Here's how the part is built. I have some questions about the finished solid (model axes, mm). A direction names the side the tool comes from. Coordinates: 2 decimals unless noted, no trailing zeros. Loops run counter-clockwise (first coordinate to the right, second up) from the corner with the lowest first, then second, coordinate; pieces in that order, holes last. Notation, with made-up numbers: M 42.25,4.5 L 74.25,4.5 A15 ccw 74.25,14.5 Z; hole C 67.25,11.5 d1. An arc over 180 degrees is marked long. Use one line per item in the form item = value. Start each with the question number.
(1) On a 3-axis mill with a long thin cutter (end or side, diameter ignored), from which of +Z, -Z, +X, -X, +Y, -Y can I reach the whole of each face in a straight line? I mean faces 4 (the flat face through (-23, 46, 27)), 5 (the flat face through (-1, 40, 34)), 6 (the flat face through (-26.5, 45, 0)), 7 (the cylindrical face through (-105, 20, -47)). Say none if no direction works.
(2) Imagine slicing it at C-C, the plane x = 46. Please give me the cut outline in (y, z), and give its area (3 significant figures).
(3) Imagine slicing it at A-A, the plane z = 10. Please give me the cut outline in (x, y), and give its area (3 significant figures).
(4) Imagine slicing it at B-B, the plane y = 20. State how many separate pieces and enclosed holes the cut face has, and give its area (3 significant figures).
(5) Will these pins go through, and if not, where does the flat tip stop? P1, Ø2, axis at x = 0, z = 65, coming from the -Y side; P2, Ø5, axis at x = 56.5, z = 16.5, coming from the -Y side; P3, Ø5, axis at y = 20, z = 50, coming from the -X side.
(6) Thinking about a two-plate mould opening in X: for faces 1 (the cylindrical face through (20.997, 42.958, -26.069)), 2 (the flat face through (-110, 24, 1)), 3 (the flat face through (-1, 43, -75)), which applies, +X half, -X half, draft (parallel to the pull), parting line (faces both ways), or undercut?
(7) Please list where these lines run through material, in increasing order: L1, parallel to Z at x = -23, y = 44; L2, parallel to Z at x = -107.5, y = 20; L3, parallel to Z at x = 0, y = 43.
```python
from build123d import *

# Parameters (mm, degrees)
PAD_DEPTH       = 75
SKETCH001_R     = 3
POCKET_DEPTH    = 110.001
FILLET_R        = 3
FILLET001_R     = 1
SKETCH002_R     = 2.1
POCKET001_DEPTH = 6
POCKET002_DEPTH = 10.001
FILLET002_R     = 1
SKETCH004_R     = 1.35
POCKET003_DEPTH = 6


with BuildPart() as part:
    # Sketch → Pad (new body, symmetric)
    with BuildSketch(Plane.XY):
        Polygon((0, 40), (-100, 40), (-100, 0), (-110, 0), (-110, 50), (0, 50), align=None)
        Polygon((0, 40), (0, 50), align=None)
    extrude(amount=PAD_DEPTH, both=True)

    # Sketch001 (on Face3 of Pad) → Pocket (cut, through all)
    with BuildSketch(Plane(origin=(-110, 0, 0), x_dir=(0, -1, 0), z_dir=(-1, 0, 0))):
        with Locations((-20, -50)):
            Circle(SKETCH001_R)
        with Locations((-20, 50)):
            Circle(SKETCH001_R)
    extrude(amount=-POCKET_DEPTH, mode=Mode.SUBTRACT)

    # Fillet
    fillet_edges = [part.edges().sort_by_distance(p)[0] for p in [
        (-105, 0, -75),
        (-100, 40, 0),
        (-105, 0, 75),
        (-110, 50, 0),
    ]]
    fillet(fillet_edges, radius=FILLET_R)

    # Fillet001
    fillet001_edges = [part.edges().sort_by_distance(p)[0] for p in [
        (-110, 25, 75),
        (-100, 0, 0),
    ]]
    fillet(fillet001_edges, radius=FILLET001_R)

    # Sketch002 (on Face1 of Fillet001) → Pocket001 (cut)
    with BuildSketch(Plane.XZ.offset(-40)):
        with Locations((-23, -26.7)):
            Circle(SKETCH002_R)
        with Locations((-23, 26.7)):
            Circle(SKETCH002_R)
    extrude(amount=-POCKET001_DEPTH, mode=Mode.SUBTRACT)

    # Sketch003 (on Face1 of Pocket001) → Pocket002 (cut, through all)
    with BuildSketch(Plane.XZ.offset(-40)):
        with BuildLine():
            Line((0, -26.7), (-19.5, -26.7))
            ThreePointArc((-19.5, -26.7), (-20.525126, -24.225126), (-23, -23.2))
            Line((-23, -23.2), (-26.5, -23.2))
            Line((-26.5, 23.2), (-26.5, -23.2))
            Line((-23, 23.2), (-26.5, 23.2))
            ThreePointArc((-23, 23.2), (-20.525126, 24.225126), (-19.5, 26.7))
            Line((-19.5, 26.7), (0, 26.7))
            Line((0, 26.7), (0, -26.7))
        make_face()
    extrude(amount=-POCKET002_DEPTH, mode=Mode.SUBTRACT)

    # Fillet002
    fillet002_edges = [part.edges().sort_by_distance(p)[0] for p in [
        (-26.5, 45, 23.2),
        (-19.5, 45, 26.7),
        (-26.5, 45, -23.2),
        (-19.5, 45, -26.7),
    ]]
    fillet(fillet002_edges, radius=FILLET002_R)

    # Mirrored: part across YZ


with BuildPart() as part_1:
    add(part.part)
    add(part.part.mirror(Plane.YZ))

    # Sketch004 (on Face24 of Mirrored) → Pocket003 (cut)
    with BuildSketch(Plane.XZ.offset(-40)):
        with Locations((0, 65)):
            Circle(SKETCH004_R)
        with Locations((0, 48.81)):
            Circle(SKETCH004_R)
    extrude(amount=-POCKET003_DEPTH, mode=Mode.SUBTRACT)


solid = part_1.part
```
Answer:
q1.face_4 = -Y
q1.face_5 = +Z, -Z, -Y
q1.face_6 = +Y, -Y
q1.face_7 = +X, -X
q2.outline = M 40,-74 A1 ccw 41,-75 L 49,-75 A1 ccw 50,-74 L 50,74 A1 ccw 49,75 L 41,75 A1 ccw 40,74 Z
q2.area = 1,500 mm²
q3.outline = M -110,1 A1 ccw -109,0 L -101,0 A1 ccw -100,1 L -100,37 A3 cw -97,40 L -26.5,40 L -26.5,50 L -107,50 A3 ccw -110,47 Z; M 26.5,40 L 97,40 A3 cw 100,37 L 100,1 A1 ccw 101,0 L 109,0 A1 ccw 110,1 L 110,47 A3 ccw 107,50 L 26.5,50 Z
q3.area = 2,470 mm²
q4.separate_pieces = 6
q4.enclosed_holes = 0
q4.area = 2,760 mm²
q5.P1 = 46
q5.P2 = 40
q5.P3 = through
q6.face_1 = undercut
q6.face_2 = -X half
q6.face_3 = draft
q7.L1 = -75 to -28.8, -24.6 to -23.2, 23.2 to 24.6, 28.8 to 75
q7.L2 = -75 to -53, -47 to 47, 53 to 75
q7.L3 = -75 to -26.7, 26.7 to 47.46, 50.16 to 63.65, 66.35 to 75
